Autodesk Inventor part; units mm, degrees
ref_plane "YZ Plane" through (0, 0, 0) normal (1, 0, 0) x (0, 1, 0)
ref_plane "XZ Plane" through (0, 0, 0) normal (0, 1, 0) x (-1, 0, 0)
ref_plane "XY Plane" through (0, 0, 0) normal (0, 0, 1) x (1, 0, 0)
sketch "Sketch1" plane through (0, 0, 0) normal (0, 0, 1) x (1, 0, 0)
  line L0 (64, 0) -> (64, 5)
  line L1 (0, 5) -> (0, 0)
  arc A0 (49, 17) -> (15, 17) centre (32, 17) ccw
  line L2 (15, 5) -> (15, 17)
  line L3 (49, 5) -> (49, 17)
  line L4 (20, 0) -> (20, 17)
  arc A1 (44, 17) -> (20, 17) centre (32, 17) ccw
  line L5 (44, 17) -> (44, 0)
  line L6 (64, 5) -> (49, 5)
  line L7 (15, 5) -> (0, 5)
  line L8 (0, 0) -> (20, 0)
  line L9 (44, 0) -> (64, 0)
  dimension "d1" = 5
  dimension "d3" = 17
  dimension "d4" = 15
  dimension "d6" = 5
  dimension "d7" = 15
  dimension "d8" = 20
extrude "Extrusion1" add sketch "Sketch1" along normal blind 15
sketch "Sketch2" plane through (0, 5, 0) normal (0, 1, 0) x (1, 0, 0)
  line L0 (15, 0) -> (0, 0)
  line L1 (64, 0) -> (49, 0)
  line L2 (0, 0) -> (0, -15)
  point P0 (7, -7.5)
  point P1 (57, -7.5)
  dimension "d18" = 50
  dimension "d19" = 7.5
  dimension "d20" = 7.5
  dimension "d21" = 7
hole "Hole1" at (7, 5, 7.5) at (57, 5, 7.5) direction (0, -1, 0) diameter 3 end through all
properties part number "U_BRACKET_2"
The model under review builds one solid part; all positions refer to its coordinate system, in mm. A direction names the side the tool comes from. Round coordinates to 2 decimals unless told otherwise and drop trailing zeros. Loops run counter-clockwise (first coordinate to the right, second up) from the corner with the lowest first, then second, coordinate; pieces in that order, holes last. Notation, with made-up numbers: (77.5, -27) -> (111.5, -27) arc R36 ccw to (111.5, 11) -> close; hole circle Ø10 at (41.25, 15). An arc over 180 degrees is marked (long way). One line per question, with ' | ' between items. Start each with the question number.
Item 1: Wall thickness on line 1 along X through (y, z) = (3, 7.5); line 2 along Z through (x, y) = (7, 3.05); line 3 along X through (y, z) = (10.5, 11): over which ranges is each line inside the solid? List them lowest first. Write a range as [from, to].
Item 2: Machinability: for faces 1 (the face through (55, 5, 7)), 2 (the face through (54, 0, 7)), 3 (the face through (9, 5, 7)), 4 (the face through (44, 9, 7)), 5 (the face through (64, 2, 7)), which of the approach directions +Z, -Z, +X, -X, +Y, -Y give a long, thin tool a straight path to every point of the face, cutting with its end or side? Answer none if there is none.
Item 3: Add section D-D, the plane z = 1.5. Write out the cut boundary in (x, y), then the cut area to 3 significant figures.
Item 4: Add section C-C, the plane y = 24. Write out the cut boundary in (x, z).
Item 5: Add section A-A, the plane z = 7.5. Write out the cut boundary in (x, y), then the cut area to 3 significant figures.
Item 6: Draft analysis for pull direction X (two halves, no side actions). For faces 6 (the face through (32, 34, 7)), 7 (the face through (55.513, 2.465, 7.305)), 8 (the face through (49, 11, 7)), state which applies: +X half, -X half, draft (parallel to the pull), parting line (faces both ways), or undercut.
Item 7: Add section B-B, the plane x = 57. Write out the cut boundary in (y, z), then the cut area to 3 significant figures.
Item 8: For pin 1 (1 mm diameter, centred on y = 16, z = 3.5, fed in from -X); pin 2 (4.5 mm diameter, centred on x = 10, z = 8, fed in from +Y); pin 3 (6 mm diameter, centred on y = 13.5, z = 8, fed in from +X), all flat-tipped, find the tip position at first contact; note any pin that passes through.
Return value:
1) line 1: x = [0, 5.5], [8.5, 20], [44, 55.5], [58.5, 64] | line 2: z = [0, 6], [9, 15] | line 3: x = [15, 20], [44, 49]
2) face 1: +Z, -Z, +X, +Y | face 2: +Z, -Z, +X, -X, -Y | face 3: +Z, -Z, -X, +Y | face 4: +Z, -Z, -Y | face 5: +Z, -Z, +X, +Y, -Y
3) outline: (0, 0) -> (20, 0) -> (20, 17) arc R12 cw to (44, 17) -> (44, 0) -> (64, 0) -> (64, 5) -> (49, 5) -> (49, 17) arc R17 ccw to (15, 17) -> (15, 5) -> (0, 5) -> close | area: 548 mm2
4) outline: (16.51, 0) -> (22.25, 0) -> (22.25, 15) -> (16.51, 15) -> close; (41.75, 0) -> (47.49, 0) -> (47.49, 15) -> (41.75, 15) -> close
5) outline: (0, 0) -> (5.5, 0) -> (5.5, 5) -> (0, 5) -> close; (8.5, 0) -> (20, 0) -> (20, 17) arc R12 cw to (44, 17) -> (44, 0) -> (55.5, 0) -> (55.5, 5) -> (49, 5) -> (49, 17) arc R17 ccw to (15, 17) -> (15, 5) -> (8.5, 5) -> close; (58.5, 0) -> (64, 0) -> (64, 5) -> (58.5, 5) -> close | area: 518 mm2
6) face 6: parting line | face 7: undercut | face 8: +X half
7) outline: (0, 0) -> (5, 0) -> (5, 6) -> (0, 6) -> close; (0, 9) -> (5, 9) -> (5, 15) -> (0, 15) -> close | area: 60.0 mm2
8) pin 1: stops at x = 15 | pin 2: stops at y = 5 | pin 3: stops at x = 49
